Read the model definition and answer for the solid it produces. Units are mm, in the model's axes. A direction names the side the tool comes from. Coordinates: 2 decimals unless noted, no trailing zeros. Order: outer loops, then holes, each group sorted by start corner. A loop starts at its lowest first (then second) coordinate and runs counter-clockwise, first axis right, second up. Notation, with made-up numbers: M 37,72 L 56,72 A25 ccw 56,108 Z; hole C -17,-4.75 d4. An arc over 180 degrees is marked long. Use a Markdown table: item, result. Add a question column.
1) Find section C-C on y = 0. Write down the section's boundary in (x, z).
2) For faces 1 (the face through (-22, 0, 22)), 2 (the face through (40.461, -9.405, 17.748)), 3 (the face through (107, 25, 22)), 4 (the face through (108, -25, 18)), 5 (the face through (78.476, -6.674, 17.748)), determine the directions among +Z, -Z, +X, -X, +Y, -Y from which every point of the face is accessible in a straight line to the end or side of a thin tool.
3) Find section A-A on z = 6. Write down the section's boundary in (x, y).
4) The mould has two halves that part along Z. Classify faces 6 (the face through (57.104, -10.282, 17.748)), 7 (the face through (132, -20, 36)), 8 (the face through (95.05, 19.93, 17.22)): released by +Z, released by -Z, zero draft, split by the parting line, or undercut.
5) Find section D-D on x = 101. Write down the section's boundary in (y, z), plus the area to 3 significant figures.
6) Each of these flat-tipped pins is pushed along its axis until it touches: pin 1 Ø7 at (x, z) = (125, 30) entering from +Y; pin 2 Ø15.5 at (x, z) = (101, 18) entering from +Y; pin 3 Ø4 at (y, z) = (-12, 29.5) entering from +X; pin 4 Ø4.5 at (y, z) = (-1, 10) entering from -X. Where does it stop, or does it pass through?
7) Find the intervals of material crossed by probe 1 along Y at (x, z) = (100, 29); probe 2 along Z at (x, y) = (101, 18); probe 3 along Y at (x, z) = (22.5, 25), in increasing order. Write a range as [from, to].
Autodesk Inventor part; units mm, degrees
ref_plane "Arbeitsebene1" through (0, 0, 18) normal (0, 0, 1) x (1, 0, 0)
ref_plane "YZ Plane" through (0, 0, 0) normal (1, 0, 0) x (0, 1, 0)
ref_plane "XZ Plane" through (0, 0, 0) normal (0, 1, 0) x (-1, 0, 0)
sketch "Skizze1" plane through (0, 0, 0) normal (0, 0, 1) x (1, 0, 0)
  line L0 (75, 25) -> (140, 25)
  line L1 (140, -25) -> (75, -25)
  line L2 (140, 15) -> (84.3835, 15)
  line L3 (140, -15) -> (84.3835, -15)
  line L4 (175.9728, 0) -> (38.8128, 0) construction
  line L5 (75, 25) -> (75, -25) construction
  arc A0 (70, 1.5) -> (84.3835, 15) centre (61.4706, 25) ccw
  line L6 (70, 1.5) -> (70, -1.5)
  arc A1 (84.3835, -15) -> (70, -1.5) centre (61.4706, -25) ccw
  line L7 (140, 25) -> (140, 15)
  line L8 (140, -15) -> (140, -25)
  arc A2 (45.8579, 30) -> (75, 25) centre (60, 25) ccw
  line L9 (45.8579, 30) -> (0, 30)
  arc A3 (75, -25) -> (45.8579, -30) centre (60, -25) ccw
  line L10 (45.8579, -30) -> (0, -30)
  arc A4 (0, 30) -> (0, -30) centre (0, 0) ccw
  line L11 (50, 2.0871) -> (50, -2.0871)
  line L12 (35.5051, -20) -> (0, -20)
  line L13 (35.5051, 20) -> (0, 20)
  arc A5 (0, 20) -> (0, -20) centre (0, 0) ccw
  line L14 (60, 25) -> (60, -25) construction
  arc A6 (35.5051, 20) -> (50, 2.0871) centre (60, 25) ccw
  arc A7 (50, -2.0871) -> (35.5051, -20) centre (60, -25) ccw
  dimension "d17" = 30
  dimension "d18" = 50
  dimension "d19" = 25
  dimension "d20" = 3
  dimension "d21" = 80
  dimension "d28" = 15
  dimension "d30" = 30
  dimension "d34" = 20
  dimension "d36" = 25
  dimension "d37" = 25
  dimension "d38" = 60
  dimension "d39" = 20
extrude "Extrusion1" add sketch "Skizze1" along normal blind 36
sketch "Skizze2" plane through (75, 25, 0) normal (0, 1, 0) x (1, 0, 0)
  line L0 (65, 0) -> (65, -36)
  line L1 (65, 0) -> (0, 0)
  point P0 (-75, 0)
  point P1 (50, -6)
  point P2 (50, -30)
  point P3 (26, -18)
  point P4 (65, -18)
  dimension "d42" = 24
  dimension "d43" = 6
  dimension "d44" = 24
  dimension "d45" = 15
hole "Bohrung1" at (125, 25, 6) at (125, 25, 30) at (101, 25, 18) direction (0, -1, 0) diameter 12 depth 50
ref_plane "Arbeitsebene1" through (0, 0, 18) normal (0, 0, 1) x (1, 0, 0)
sketch "Skizze3" plane through (0, 0, 18) normal (0, 0, 1) x (1, 0, 0)
  arc A0 (0, 30) -> (0, -30) centre (0, 0) ccw
  arc A1 (0, 30) -> (0, -30) centre (0, 0) ccw
  line L0 (0, -30) -> (0, 30)
  dimension "d54" = 30
extrude "Extrusion2" cut sketch "Skizze3" along normal mid plane 8
equation "\"d37\" = d36"
properties part number "drawing" material "Stahl, galvanisiert"
Check result:
| question | item | result |
|---|---|---|
| 1 | outline | M -30,0 L -20,0 L -20,14 L -30,14 Z; M -30,22 L -20,22 L -20,36 L -30,36 Z; M 50,0 L 70,0 L 70,36 L 50,36 Z |
| 2 | face 1 | -X, +Y, -Y |
| 2 | face 2 | +Z, -Z |
| 2 | face 3 | +Z, -Z, +X, +Y |
| 2 | face 4 | +Z, -Z, +X, -Y |
| 2 | face 5 | +Z, -Z, +X |
| 3 | outline | M 0,-30 L 45.86,-30 A15 cw long 75,-25 L 119,-25 L 119,-15 L 84.38,-15 A25 ccw 70,-1.5 L 70,1.5 A25 ccw 84.38,15 L 119,15 L 119,25 L 75,25 A15 cw long 45.86,30 L 0,30 A30 ccw Z; M 131,-25 L 140,-25 L 140,-15 L 131,-15 Z; M 131,15 L 140,15 L 140,25 L 131,25 Z; hole M 0,-20 L 35.51,-20 A25 cw 50,-2.09 L 50,2.09 A25 cw 35.51,20 L 0,20 A20 ccw Z |
| 4 | face 6 | zero draft |
| 4 | face 7 | released by +Z |
| 4 | face 8 | undercut |
| 5 | outline | M -25,0 L -15,0 L -15,12 L -25,12 Z; M -25,24 L -15,24 L -15,36 L -25,36 Z; M 15,0 L 25,0 L 25,12 L 15,12 Z; M 15,24 L 25,24 L 25,36 L 15,36 Z |
| 5 | area | 480 mm2 |
| 6 | pin 1 | passes through |
| 6 | pin 2 | stops at y = 25 |
| 6 | pin 3 | stops at x = 83.92 |
| 6 | pin 4 | stops at x = -30 |
| 7 | probe 1 | y = [-25, -15], [15, 25] |
| 7 | probe 2 | z = [0, 12], [24, 36] |
| 7 | probe 3 | y = [-30, -20], [20, 30] |
